```python
from build123d import *

# Parameters (mm, degrees)
SKETCH1_R           = 29.175
SKETCH1_R_2         = 4
BOSS_EXTRUDE1_DEPTH = 44.5
FILLET1_R           = 20
SKETCH2_R           = 11
CUT_EXTRUDE1_DEPTH  = 10


with BuildPart() as part:
    # Sketch1 → Boss-Extrude1 (new body)
    with BuildSketch(Plane(origin=(0, 0, 0), x_dir=(1, 0, 0), z_dir=(0, 1, 0))):
        with Locations(Location((0, 0, 0), (0, 0, 270))):
            Circle(SKETCH1_R)
        with Locations(Location((0, 0, 0), (0, 0, 270))):
            Circle(SKETCH1_R_2, mode=Mode.SUBTRACT)
    extrude(amount=BOSS_EXTRUDE1_DEPTH)

    # Fillet1
    fillet1_edges = [part.edges().sort_by_distance(p)[0] for p in [
        (0, 44.5, -4),
    ]]
    fillet(fillet1_edges, radius=FILLET1_R)

    # Sketch2 → Cut-Extrude1 (cut)
    with BuildSketch(Plane.XZ):
        with Locations(Location((0, 0, 0), (0, 0, 270))):
            Circle(SKETCH2_R)
    extrude(amount=-CUT_EXTRUDE1_DEPTH, mode=Mode.SUBTRACT)


solid = part.part
```
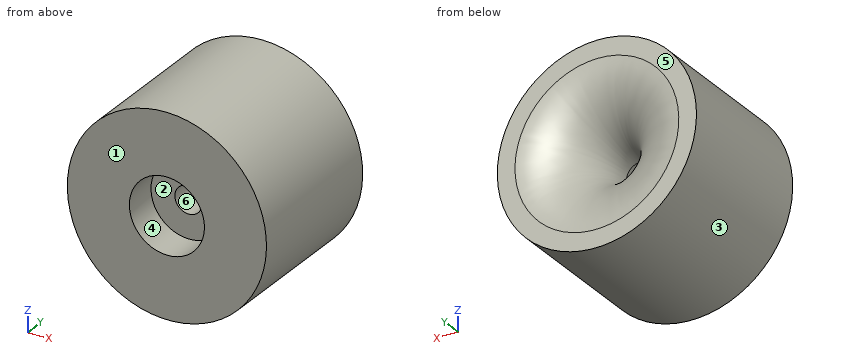
CAD build for the part. Positions are in the model's coordinates, mm. Face numbers are marked on the shaded views. A direction names the side the tool comes from. Coordinates: 2 decimals unless noted, no trailing zeros. Order: outer loops, then holes, each group sorted by start corner. A loop starts at its lowest first (then second) coordinate and runs counter-clockwise, first axis right, second up.
(1) Drill centre lines: L1, parallel to X at y = 21.75, z = 0 (3 decimals); L2, parallel to X at y = 6.5, z = 0 (3 decimals); L3, parallel to Y at x = -17.5, z = -1.5. Where is each one in solid material? Low to high.
Solution:
L1: x = -29.175 to -4, 4 to 29.175
L2: x = -29.175 to -11, 11 to 29.175
L3: y = 0 to 43.44
(2) Saw through at A-A, the plane z = 0. Write the cut outline in (x, y) (3 decimals), and give its area (3 significant figures).
Solution:
outline: (-29.175, 0) - (-11, 0) - (-11, 10) - (-4, 10) - (-4, 24.5) arc R20 ccw to (-24, 44.5) - (-29.175, 44.5) - close; (4, 10) - (11, 10) - (11, 0) - (29.175, 0) - (29.175, 44.5) - (24, 44.5) arc R20 ccw to (4, 24.5) - close
area: 1,930 mm2
(3) Pin check, flat tips, straight feed: pin 1 Ø6.5 at (x, z) = (0, 0) entering from +Y; pin 2 Ø2 at (x, y) = (6.5, 26) entering from +Z; pin 3 Ø6 at (x, y) = (13, 36) entering from -Z; pin 4 Ø1.5 at (y, z) = (18.5, -12.5) entering from +X. Stop position of each tip, or through.
Solution:
pin 1: passes through
pin 2: stops at z = 28.65
pin 3: stops at z = -27.41
pin 4: stops at x = 26.7
(4) Mould opens along X. For the marked faces 3, 4, 5 and 6 say: released by +X, released by -X, zero draft, split by the parting line, or undercut.
Solution:
face 3: split by the parting line
face 4: undercut
face 5: zero draft
face 6: undercut
(5) Saw through at D-D, the plane y = 31.5. Write the cut outline in (x, z) (3 decimals), and give its area (3 significant figures).
Solution:
outline: circle Ø58.35 at (0, 0); hole circle Ø10.53 at (0, 0)
area: 2,590 mm2
(6) Which spindle directions (+Z, -Z, +X, -X, +Y, -Y) get a long thin tool onto all of the face, cutting with end or side? Do the marked faces 1 and 2. Say none if no direction does.
Solution:
face 1: +Z, -Z, +X, -X, -Y
face 2: -Y
(7) Saw through at C-C, the plane y = 16. Write the cut outline in (x, z) (3 decimals).
Solution:
outline: circle Ø58.35 at (0, 0); hole circle Ø8 at (0, 0)
(8) Saw through at B-B, the plane x = 0. Write the cut outline in (y, z) (3 decimals).
Solution:
outline: (0, -29.175) - (44.5, -29.175) - (44.5, -24) arc R20 ccw to (24.5, -4) - (10, -4) - (10, -11) - (0, -11) - close; (0, 11) - (10, 11) - (10, 4) - (24.5, 4) arc R20 ccw to (44.5, 24) - (44.5, 29.175) - (0, 29.175) - close
